from build123d import *

# Parameters (mm, degrees)
F0_W     = 204.3
F0_H     = 114.3
F0_R     = 14
F1_DEPTH = 10
F2_DEPTH = 1.5
F4_D     = 4


with BuildPart() as f1:
    # F0 (on Top) → F1 (new body)
    with BuildSketch(Plane.XY):
        Rectangle(F0_W, F0_H)
        with Locations((-57.15, 0)):
            Circle(F0_R, mode=Mode.SUBTRACT)
        Circle(F0_R, mode=Mode.SUBTRACT)
        with Locations((-57.15, 0)):
            Circle(F0_R)
        Circle(F0_R)
    extrude(amount=F1_DEPTH)

    # F0 (on Top) → F2 (join)
    with BuildSketch(Plane.XY):
        with Locations((-57.15, 0)):
            Circle(F0_R)
        Circle(F0_R)
    extrude(amount=-F2_DEPTH)

    # F4 (through all)
    with Locations(Plane(origin=(0, 0, -1.5), x_dir=(1, 0, 0), z_dir=(0, 0, -1))):
        with Locations((-57.15, 0), (0, 0)):
            Hole(F4_D / 2)


solid = f1.part
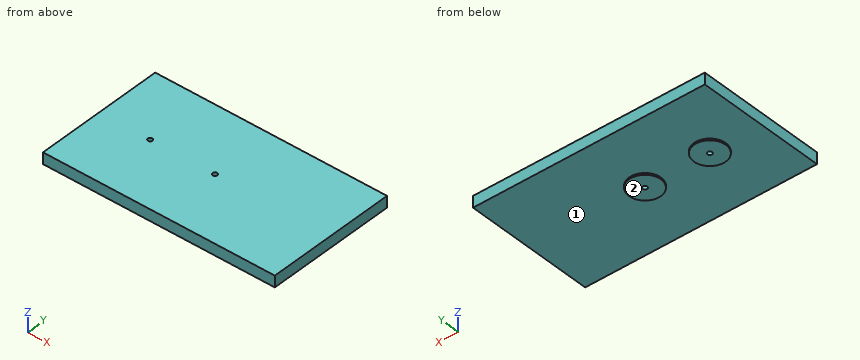
Work out the finished part from the listing and answer in its coordinate system (mm). Face numbers are marked on the shaded views. A direction names the side the tool comes from. Coordinates: 2 decimals unless noted, no trailing zeros. Write each loop counter-clockwise with the first axis right and the second up, starting at its lowest first coordinate (ties: lowest second). Pieces come first, ordered by that corner, then holes. Notation, with made-up numbers: (33, -5.75) - (61, -5.75) arc R8 ccw to (61, 1.25) - close; hole circle Ø1 at (66.25, 54.25). An arc over 180 degrees is marked (long way). One line per question, with ' | ' between items.
1) Find section B-B, the plane x = -57.15. Determine the outline of the cut face in (y, z), and give its area (3 significant figures).
Checks:
outline: (-57.15, 0) - (-14, 0) - (-14, -1.5) - (-2, -1.5) - (-2, 10) - (-57.15, 10) - close; (2, -1.5) - (14, -1.5) - (14, 0) - (57.15, 0) - (57.15, 10) - (2, 10) - close | area: 1,140 mm2
2) Find section A-A, the plane y = 0. Determine the outline of the cut face in (x, z), and give its area (4 significant figures).
Checks:
outline: (-102.15, 0) - (-71.15, 0) - (-71.15, -1.5) - (-59.15, -1.5) - (-59.15, 10) - (-102.15, 10) - close; (-55.15, -1.5) - (-43.15, -1.5) - (-43.15, 0) - (-14, 0) - (-14, -1.5) - (-2, -1.5) - (-2, 10) - (-55.15, 10) - close; (2, -1.5) - (14, -1.5) - (14, 0) - (102.15, 0) - (102.15, 10) - (2, 10) - close | area: 2,035 mm2
3) For the marked faces 1 and 2, determine the directions among +Z, -Z, +X, -X, +Y, -Y from which every point of the face is accessible in a straight line to the end or side of a thin tool.
Checks:
face 1: -Z | face 2: -Z, +X, -X, +Y, -Y
4) A flat-ended cylindrical pin translates along its axis: P1, Ø10, axis at x = 55, y = -33, coming from the -Z side. Find the tip coordinate at first contact, or state that the pin passes through.
Checks:
P1: z = 0
5) Find section D-D, the plane x = -82.5. Determine the outline of the cut face in (y, z).
Checks:
outline: (-57.15, 0) - (57.15, 0) - (57.15, 10) - (-57.15, 10) - close
6) Consider probe 1 along Y at (x, z) = (0, 7); probe 2 along Z at (x, y) = (-29, -23.5). Determine where each line is inside the solid, lowest interval first. Write a range as [from, to].
Checks:
probe 1: [-57.15, -2], [2, 57.15] | probe 2: [0, 10]
7) Find section C-C, the plane y = 37. Determine the outline of the cut face in (x, z), and give its area (3 significant figures).
Checks:
outline: (-102.15, 0) - (102.15, 0) - (102.15, 10) - (-102.15, 10) - close | area: 2,040 mm2
